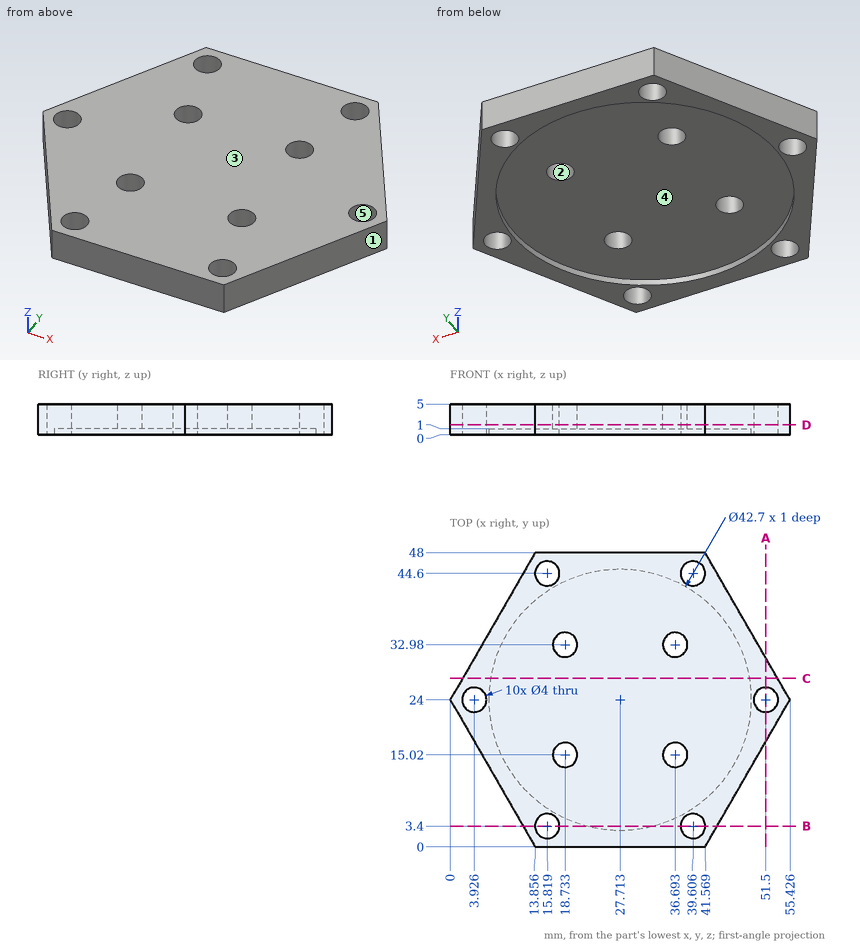
Geometry check sheet. Reference: drawing and pictorial views, mm from the part's lowest x, y, z. A direction names the side the tool comes from. Give positions to 0.01 mm unless a question says otherwise; leave off trailing zeros. Write each loop counter-clockwise with the first axis right and the second up, starting at its lowest first coordinate (ties: lowest second). Pieces come first, ordered by that corner, then holes. Notation, with made-up numbers: M 61,24.25 L 113,24.25 A21 ccw 113,58.25 Z; hole C 57.5,72.5 d3. An arc over 180 degrees is marked long. Answer as CSV lines item,"result". Start each with the question number.
Q1. Section check D-D, the plane z = 1.6. Give the number of separate pieces and of enclosed holes in the cut face, then the cut area to 3 significant figures.
Q2. Section check C-C, the plane y = 27.5. Record the cut outline in (x, z) (1 decimal).
Q3. Material ranges on L1, parallel to Y at x = 16, z = 3.1; L2, parallel to Y at x = 20, z = 1.5 (1 decimal); L3, parallel to X at y = 45.5, z = 0.6 (1 decimal), recorded low to high.
Q4. Go/stop test with flat-tipped pins: pin 1 (3.5 mm diameter, centred on x = 18.73, y = 15.02, fed in from +Z); pin 2 (13 mm diameter, centred on x = 35, y = 17, fed in from -Z). Record where each tip stops, or that it passes through.
Q5. Release check for a two-part mould opening along X. For the marked faces 1, 2 and 3 record: pulls with the +X half, pulls with the -X half, needs draft (parallel to the pull), parting line crosses it, or undercut.
Q6. Section check B-B, the plane y = 3.4. Record the cut outline in (x, z), then the cut area to 3 significant figures.
Q7. Tool access check on the marked faces 4 and 5. Record the directions out of +Z, -Z, +X, -X, +Y, -Y that give a thin tool (end or side, any length) a straight path to the whole face; none if there is none.
Q8. Section check A-A, the plane x = 51.5. Record the cut outline in (y, z), then the cut area to 3 significant figures.
Geometry says:
1,separate pieces,"1"
1,enclosed holes,"10"
1,area,"1,870 mm^2"
2,outline,"M 2,0 L 6.7,0 L 6.7,1 L 48.8,1 L 48.8,0 L 53.4,0 L 53.4,5 L 2,5 Z"
3,L1,"0 to 1.41, 5.39 to 42.61, 46.59 to 48"
3,L2,"0 to 13.5, 16.6 to 31.4, 34.5 to 48"
3,L3,"12.4 to 14, 17.6 to 37.8, 41.4 to 43"
4,pin 1,"through"
4,pin 2,"z = 1"
5,face 1,"pulls with the +X half"
5,face 2,"undercut"
5,face 3,"needs draft"
6,outline,"M 11.89,0 L 13.82,0 L 13.82,5 L 11.89,5 Z; M 17.82,0 L 22.1,0 L 22.1,1 L 33.32,1 L 33.32,0 L 37.61,0 L 37.61,5 L 17.82,5 Z; M 41.61,0 L 43.53,0 L 43.53,5 L 41.61,5 Z"
6,area,"107 mm^2"
7,face 4,"-Z"
7,face 5,"+Z, -Z"
8,outline,"M 17.2,0 L 22,0 L 22,5 L 17.2,5 Z; M 26,0 L 30.8,0 L 30.8,5 L 26,5 Z"
8,area,"48.0 mm^2"
